from build123d import *

# Parameters (mm, degrees)
BOSS_EXTRUDE2_DEPTH      = 6
SKETCH2_R                = 4
SKETCH2_W                = 30
SKETCH2_H                = 8.3
CUT_EXTRUDE1_DEPTH       = 341.487943986
CROQUIS1_W               = 103.610606389
CROQUIS1_H               = 1.56
SALIENTE_EXTRUIR2_DEPTH  = 6
SALIENTE_EXTRUIR3_DEPTH  = 6
SALIENTE_EXTRUIR4_START  = -6
SALIENTE_EXTRUIR4_DEPTH  = 6
SALIENTE_EXTRUIR5_DEPTH  = 6
SALIENTE_EXTRUIR6_DEPTH  = 6
CROQUIS7_W               = 103.610606389
CROQUIS7_H               = 0.56
SALIENTE_EXTRUIR7_DEPTH  = 6
SALIENTE_EXTRUIR8_DEPTH  = 6
SKETCH3_R                = 1.5
CUT_EXTRUDE2_DEPTH       = 341.487943986
CUT_EXTRUDE3_DEPTH       = 341.487943986
CROQUIS9_W               = 152
CROQUIS9_H               = 0.3
CORTAR_EXTRUIR1_DEPTH    = 10
CORTAR_EXTRUIR2_DEPTH    = 6
CROQUIS14_W              = 17
CROQUIS14_H              = 12
CORTAR_EXTRUIR4_DEPTH    = 10
CROQUIS15_R              = 4
CORTAR_EXTRUIR5_DEPTH    = 10
SALIENTE_EXTRUIR10_DEPTH = 6
SALIENTE_EXTRUIR11_DEPTH = 6
CROQUIS18_W              = 98.157526679
CROQUIS18_H              = 1.5
CORTAR_EXTRUIR6_DEPTH    = 6


with BuildPart() as part:
    # Sketch1 → Boss-Extrude2 (new body)
    with BuildSketch(Plane.XY):
        with BuildLine():
            Line((0, 0), (-220, 0))
            Line((-220, 0), (-220, 71.45))
            Line((-220, 71.45), (-116.389393611, 71.45))
            ThreePointArc((-116.389393611, 71.45), (-107.149394721, 74.662079518), (-101.894274329, 82.913063942))
            Line((-101.894274329, 82.913063942), (-60, 259.8))
            Line((-60, 259.8), (0, 259.8))
            Line((0, 259.8), (0, 0))
        make_face()
    extrude(amount=BOSS_EXTRUDE2_DEPTH)

    # Sketch2 → Cut-Extrude1 (cut, through all)
    with BuildSketch(Plane.XY.offset(6)):
        with Locations((-205, 36.3)):
            Circle(SKETCH2_R)
        with Locations((-24.8, 244.8)):
            Circle(SKETCH2_R)
        with Locations((-24.8, 125)):
            Circle(SKETCH2_R)
        with Locations((-80, 36.3)):
            Circle(SKETCH2_R)
        with Locations((-205, 4.15)):
            Rectangle(SKETCH2_W, SKETCH2_H)
        Polygon((-38, 0), (-38, 19), (-10.7, 46.3), (0, 46.3), (0, 0), align=None)
    extrude(amount=-CUT_EXTRUDE1_DEPTH, mode=Mode.SUBTRACT)

    # Croquis1 → Saliente-Extruir2 (add)
    with BuildSketch(Plane.XY.offset(6)):
        with Locations((-168.194696806, 72.23)):
            Rectangle(CROQUIS1_W, CROQUIS1_H)
    extrude(amount=-SALIENTE_EXTRUIR2_DEPTH)

    # Croquis3 → Saliente-Extruir3 (add)
    with BuildSketch(Plane.XY.offset(6)):
        Polygon((-101.894274329, 82.913063942), (-103.412279578, 83.272591501), (-60, 259.8), align=None)
    extrude(amount=-SALIENTE_EXTRUIR3_DEPTH)

    # Croquis4 → Saliente-Extruir4 (add)
    with BuildSketch(Plane.XY.offset(6).offset(SALIENTE_EXTRUIR4_START)):
        with BuildLine():
            Line((-103.412279578, 83.272591501), (-101.894274329, 82.913063942))
            ThreePointArc((-101.894274329, 82.913063942), (-107.149394721, 74.662079518), (-116.389393611, 71.45))
            Line((-116.389393611, 71.45), (-116.389393611, 73.01))
            ThreePointArc((-116.389393611, 73.01), (-108.117056079, 75.88569363), (-103.412279578, 83.272591501))
        make_face()
    extrude(amount=SALIENTE_EXTRUIR4_DEPTH)

    # Croquis5 → Saliente-Extruir5 (add)
    with BuildSketch(Plane.XY.offset(6)):
        Polygon((-105, 102.74), (-55, 102.74), (-103.412279578, 83.272591501), align=None)
    extrude(amount=-SALIENTE_EXTRUIR5_DEPTH)

    # Croquis6 → Saliente-Extruir6 (add)
    with BuildSketch(Plane.XY.offset(6)):
        Polygon((-98.157526679, 104.64), (-105.154959958, 104.64), (-105, 102.74), (-98.624781775, 102.74), align=None)
    extrude(amount=-SALIENTE_EXTRUIR6_DEPTH)

    # Croquis7 → Saliente-Extruir7 (add)
    with BuildSketch(Plane.XY.offset(6)):
        with Locations((-168.194696806, 73.29)):
            Rectangle(CROQUIS7_W, CROQUIS7_H)
    extrude(amount=-SALIENTE_EXTRUIR7_DEPTH)

    # Croquis8 → Saliente-Extruir8 (add)
    with BuildSketch(Plane.XY.offset(6)):
        with BuildLine():
            Line((-116.389393611, 73.57), (-117.98880457, 71.652693326))
            Line((-117.98880457, 71.652693326), (-105.380568296, 73.057716723))
            Line((-105.380568296, 73.057716723), (-100.684832206, 83.373546401))
            Line((-100.684832206, 83.373546401), (-103.622774874, 85.853523162))
            ThreePointArc((-103.622774874, 85.853523162), (-107.531184208, 77.13952683), (-116.389393611, 73.57))
        make_face()
    extrude(amount=-SALIENTE_EXTRUIR8_DEPTH)

    # Sketch3 → Cut-Extrude2 (cut, through all)
    with BuildSketch(Plane.XY.offset(6)):
        with Locations((-202.75, 62.07)):
            Circle(SKETCH3_R)
        with Locations((-129.75, 62.07)):
            Circle(SKETCH3_R)
    extrude(amount=-CUT_EXTRUDE2_DEPTH, mode=Mode.SUBTRACT)

    # Sketch4 → Cut-Extrude3 (cut, through all)
    with BuildSketch(Plane.XY.offset(6)):
        with BuildLine():
            Line((-103.622774874, 85.853523162), (-103.622774874, 78.57))
            ThreePointArc((-103.622774874, 78.57), (-105.087240968, 75.034466094), (-108.622774874, 73.57))
            Line((-108.622774874, 73.57), (-116.389393611, 73.57))
            ThreePointArc((-116.389393611, 73.57), (-107.531184208, 77.13952683), (-103.622774874, 85.853523162))
        make_face()
    extrude(amount=-CUT_EXTRUDE3_DEPTH, mode=Mode.SUBTRACT)

    # Croquis9 → Cortar-Extruir1 (cut)
    with BuildSketch(Plane.XY.offset(6)):
        with Locations((-114, 0.15)):
            Rectangle(CROQUIS9_W, CROQUIS9_H)
    extrude(amount=-CORTAR_EXTRUIR1_DEPTH, mode=Mode.SUBTRACT)

    # Croquis11 → Cortar-Extruir2 (cut)
    with BuildSketch(Plane.XY.offset(6)):
        Polygon((-10.7, 46.3), (-19.7, 46.3), (-38, 28), (-38, 19), align=None)
    extrude(amount=-CORTAR_EXTRUIR2_DEPTH, mode=Mode.SUBTRACT)

    # Croquis14 → Cortar-Extruir4 (cut)
    with BuildSketch(Plane.XY.offset(6)):
        with Locations((-8.5, 159.05)):
            Rectangle(CROQUIS14_W, CROQUIS14_H)
    extrude(amount=-CORTAR_EXTRUIR4_DEPTH, mode=Mode.SUBTRACT)

    # Croquis15 → Cortar-Extruir5 (cut)
    with BuildSketch(Plane.XY.offset(6)):
        with Locations((-80, 41.8)):
            Circle(CROQUIS15_R)
    extrude(amount=-CORTAR_EXTRUIR5_DEPTH, mode=Mode.SUBTRACT)

    # Croquis16 → Saliente-Extruir10 (add)
    with BuildSketch(Plane.XY.offset(6)):
        with BuildLine():
            ThreePointArc((-77.09526249, 39.05), (-80, 37.8), (-82.90473751, 39.05))
            ThreePointArc((-82.90473751, 39.05), (-80, 32.3), (-77.09526249, 39.05))
        make_face()
    extrude(amount=-SALIENTE_EXTRUIR10_DEPTH)

    # Croquis17 → Saliente-Extruir11 (add)
    with BuildSketch(Plane.XY.offset(6)):
        Polygon((-98.157526679, 104.64), (-98.157526679, 259.8), (-60, 259.8), align=None)
    extrude(amount=-SALIENTE_EXTRUIR11_DEPTH)

    # Croquis18 → Cortar-Extruir6 (cut)
    with BuildSketch(Plane.XY.offset(6)):
        with Locations((-49.07876334, 259.05)):
            Rectangle(CROQUIS18_W, CROQUIS18_H)
    extrude(amount=-CORTAR_EXTRUIR6_DEPTH, mode=Mode.SUBTRACT)


solid = part.part
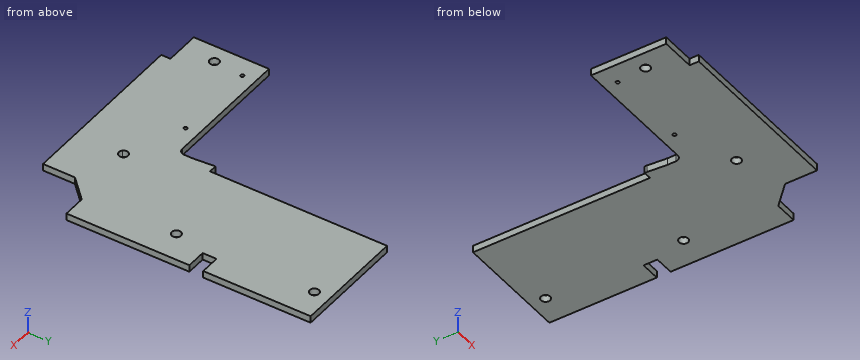
Could you check a few things on this model? Use its own coordinates, in mm. Round coordinates to 2 decimals unless told otherwise and drop trailing zeros. Order: outer loops, then holes, each group sorted by start corner. A loop starts at its lowest first (then second) coordinate and runs counter-clockwise, first axis right, second up.
(1) Imagine slicing it at C-C (x = -24.8). Write out the boundary of the cut face in (y, z), plus the area to 3 significant figures.
Response values:
outline: (41.2, 0) - (121, 0) - (121, 6) - (41.2, 6) - close; (129, 0) - (240.8, 0) - (240.8, 6) - (129, 6) - close; (248.8, 0) - (258.3, 0) - (258.3, 6) - (248.8, 6) - close
area: 1,210 mm2
(2) Imagine slicing it at A-A (x = -80). Write out the boundary of the cut face in (y, z).
Response values:
outline: (0.3, 0) - (37.8, 0) - (37.8, 6) - (0.3, 6) - close; (45.8, 0) - (258.3, 0) - (258.3, 6) - (45.8, 6) - close
(3) Imagine slicing it at D-D (z = 2.5). Write out the boundary of the cut face in (x, y).
Response values:
outline: (-220, 8.3) - (-190, 8.3) - (-190, 0.3) - (-38, 0.3) - (-38, 28) - (-19.7, 46.3) - (0, 46.3) - (0, 153.05) - (-17, 153.05) - (-17, 165.05) - (0, 165.05) - (0, 258.3) - (-98.16, 258.3) - (-98.16, 104.64) - (-105.15, 104.64) - (-103.62, 85.85) - (-103.62, 78.57) arc R5 cw to (-108.62, 73.57) - (-220, 73.57) - close; hole circle Ø8 at (-205, 36.3); hole circle Ø3 at (-202.75, 62.07); hole circle Ø3 at (-129.75, 62.07); hole circle Ø8 at (-80, 41.8); hole circle Ø8 at (-24.8, 125); hole circle Ø8 at (-24.8, 244.8)
(4) Please list where these lines run through material, in increasing order: line 1 along Y through (x, z) = (-205, 2.9); line 2 along X through (y, z) = (38.5, 3.6); line 3 along Y through (x, z) = (-24.8, 3.6).
Response values:
line 1: y = 8.3 to 32.3, 40.3 to 73.57
line 2: x = -220 to -208.34, -201.66 to -82.26, -77.74 to -27.5
line 3: y = 41.2 to 121, 129 to 240.8, 248.8 to 258.3
(5) I'm going to push flat-ended pins straight in: pin 1 (1.8 mm diameter, centred on y = 160.5, z = 3, fed in from +X); pin 2 (1.8 mm diameter, centred on x = -101.5, z = 2.5, fed in from +Y); pin 3 (3 mm diameter, centred on y = 145.5, z = 4.5, fed in from -X); pin 4 (10 mm diameter, centred on x = -105, y = 162.5, fed in from -Z). Where does each tip first touch, or does it pass through?
Response values:
pin 1: stops at x = -17
pin 2: stops at y = 104.64
pin 3: stops at x = -98.16
pin 4: passes through
(6) Imagine slicing it at B-B (y = 125). Write out the boundary of the cut face in (x, z).
Response values:
outline: (-98.16, 0) - (-28.8, 0) - (-28.8, 6) - (-98.16, 6) - close; (-20.8, 0) - (0, 0) - (0, 6) - (-20.8, 6) - close
